Autodesk Inventor part; units mm, degrees
ref_plane "YZ Plane" through (0, 0, 0) normal (1, 0, 0) x (0, 1, 0)
ref_plane "XZ Plane" through (0, 0, 0) normal (0, 1, 0) x (-1, 0, 0)
ref_plane "XY Plane" through (0, 0, 0) normal (0, 0, 1) x (1, 0, 0)
sketch "Sketch1" plane through (0, 0, 0) normal (1, 0, 0) x (0, 1, 0)
  line L0 (95.25, 812.8) -> (44.45, 812.8) construction
  line L1 (44.45, 812.8) -> (44.45, 0) construction
  line L2 (44.45, 0) -> (95.25, 0) construction
  line L3 (95.25, 0) -> (95.25, 812.8) construction
  line L4 (95.25, 0) -> (44.45, 0) construction
  line L5 (44.45, 25.4) -> (95.25, 25.4) construction
  circle A0 centre (190.5, 0) radius 50.8 construction
  circle A1 centre (95.25, 279.4) radius 25.4 construction
  circle A2 centre (274.9493, 279.9916) radius 9.525 construction
  circle A3 centre (274.9493, 279.9916) radius 25.4 construction
  circle A4 centre (274.9493, 279.9916) radius 31.75 construction
  circle A5 centre (609.6, 438.15) radius 50.8 construction
  circle A6 centre (274.9493, 279.9916) radius 30.48 construction
  circle A7 centre (587.8333, 365.125) radius 25.4 construction
  circle A8 centre (587.8333, 511.175) radius 25.4 construction
  line L6 (587.8333, 485.775) -> (587.8333, 390.525) construction
  circle A9 centre (490.3356, 512.7625) radius 14.351
  circle A10 centre (392.825, 512.7625) radius 14.351
  circle A11 centre (490.3356, 363.5375) radius 14.351
  line L7 (587.8333, 511.175) -> (490.3356, 512.7625) construction
  line L8 (587.8333, 365.125) -> (490.3356, 363.5375) construction
  circle A12 centre (490.3356, 512.7625) radius 25.4 construction
  circle A13 centre (490.3356, 363.5375) radius 25.4 construction
  line L9 (490.3356, 487.3625) -> (490.3356, 388.9375) construction
  circle A14 centre (392.825, 512.7625) radius 25.4 construction
  circle A15 centre (392.825, 363.5375) radius 25.4 construction
  circle A16 centre (392.825, 363.5375) radius 14.351
  line L10 (490.3356, 512.7625) -> (392.825, 512.7625) construction
  line L11 (490.3356, 363.5375) -> (392.825, 363.5375) construction
  line L12 (392.825, 487.3625) -> (392.825, 388.9375) construction
  circle A17 centre (295.3189, 511.8309) radius 25.4 construction
  circle A18 centre (295.3189, 362.6059) radius 25.4 construction
  circle A19 centre (203.1597, 479.9719) radius 25.4 construction
  circle A20 centre (295.3189, 511.8309) radius 14.351
  circle A21 centre (295.3189, 362.6059) radius 14.351
  circle A22 centre (203.1597, 479.9719) radius 14.351
  line L13 (392.825, 512.7625) -> (295.3189, 511.8309) construction
  line L14 (392.825, 363.5375) -> (295.3189, 362.6059) construction
  line L15 (295.3189, 486.4309) -> (295.3189, 388.0059) construction
  line L16 (295.3189, 511.8309) -> (203.1597, 479.9719) construction
  circle A23 centre (123.1487, 424.2353) radius 25.4 construction
  circle A24 centre (123.1487, 424.2353) radius 14.351
  line L17 (203.1597, 479.9719) -> (123.1487, 424.2353) construction
  circle A25 centre (95.25, 279.4) radius 14.351
  line L18 (609.6, 355.6) -> (44.45, 355.6) construction
  line L19 (44.45, 355.6) -> (44.45, 330.2) construction
  line L20 (44.45, 330.2) -> (609.6, 330.2) construction
  line L21 (609.6, 330.2) -> (609.6, 355.6) construction
  line L22 (95.25, 241.3) -> (44.45, 241.3) construction
  line L23 (44.45, 241.3) -> (44.45, 215.9) construction
  line L24 (44.45, 215.9) -> (95.25, 215.9) construction
  line L25 (95.25, 215.9) -> (95.25, 241.3) construction
  circle A26 centre (244.475, 279.4) radius 25.4 construction
  circle A27 centre (244.475, 279.4) radius 14.351
  line L26 (218.8463, 459.9947) -> (279.6322, 382.5831) construction
  circle A28 centre (274.9493, 279.9916) radius 8.89 construction
  circle A29 centre (288.401, 252.6405) radius 21.59 construction
  circle A30 centre (244.475, 279.4) radius 21.59 construction
  circle A31 centre (288.401, 252.6405) radius 14.351
  circle A32 centre (587.8333, 511.175) radius 14.351
  circle A33 centre (587.8333, 365.125) radius 14.351
  line L27 (95.25, 647.7) -> (609.6, 647.7) construction
  line L28 (609.6, 647.7) -> (609.6, 622.3) construction
  line L29 (609.6, 622.3) -> (95.25, 622.3) construction
  line L30 (95.25, 622.3) -> (95.25, 647.7) construction
  circle A34 centre (600.5333, 552.45) radius 3.2639
  circle A35 centre (600.5333, 552.45) radius 6.35 construction
  circle A36 centre (600.5333, 336.55) radius 3.2639
  circle A37 centre (600.5333, 336.55) radius 6.35 construction
  circle A38 centre (114.3, 552.45) radius 3.2639
  circle A39 centre (114.3, 552.45) radius 6.35 construction
  line L31 (595.3031, 535.4518) -> (598.6659, 546.3808) construction
  circle A40 centre (63.5, 264.8503) radius 3.2639
  circle A41 centre (63.5, 264.8503) radius 6.35 construction
  line L32 (337.9424, 330.2) -> (600.5333, 330.2)
  circle A42 centre (288.401, 252.6405) radius 24.13 construction
  circle A43 centre (244.475, 279.4) radius 24.13 construction
  line L33 (72.1591, 268.8184) -> (69.2727, 267.4957) construction
  line L34 (609.6, 342.9) -> (44.45, 342.9) construction
  line L35 (265.0822, 266.8462) -> (267.7937, 265.1944) construction
  circle A44 centre (318.8924, 273.2978) radius 3.2639
  circle A45 centre (253.4257, 241.1003) radius 3.2639
  line L36 (95.25, 558.8) -> (44.45, 558.8) construction
  line L37 (44.45, 558.8) -> (44.45, 533.4) construction
  line L38 (44.45, 533.4) -> (95.25, 533.4) construction
  line L39 (95.25, 533.4) -> (95.25, 558.8) construction
  line L40 (114.3, 558.8) -> (600.5333, 558.8)
  line L41 (108.0468, 553.5545) -> (57.2468, 265.9549)
  line L42 (285.1949, 228.7245) -> (62.6563, 258.5566)
  circle A46 centre (318.8924, 273.2978) radius 6.35 construction
  circle A47 centre (253.4257, 241.1003) radius 6.35 construction
  arc A48 (114.3, 558.8) -> (108.0468, 553.5545) centre (114.3, 552.45) ccw
  arc A49 (57.2468, 265.9549) -> (62.6563, 258.5566) centre (63.5, 264.8503) ccw
  line L43 (312.6148, 274.2541) -> (306.3372, 275.2103) construction
  line L44 (313.6352, 269.7362) -> (308.3781, 266.1746) construction
  line L45 (259.4559, 243.09) -> (265.4861, 245.0797) construction
  line L46 (256.5005, 246.6562) -> (259.5753, 252.2121) construction
  line L47 (325.2424, 317.5) -> (325.2424, 273.2978)
  arc A50 (337.9424, 330.2) -> (325.2424, 317.5) centre (337.9424, 317.5) ccw
  line L48 (324.5494, 270.4133) -> (309.8976, 241.6792)
  arc A51 (324.5494, 270.4133) -> (325.2424, 273.2978) centre (318.8924, 273.2978) ccw
  arc A52 (285.1949, 228.7245) -> (309.8976, 241.6792) centre (288.401, 252.6405) ccw
  circle A53 centre (431.8, 342.9) radius 3.2639
  circle A54 centre (457.2, 342.9) radius 3.2639
  circle A55 centre (520.7, 342.9) radius 3.2639
  circle A56 centre (546.1, 342.9) radius 3.2639
  line L49 (606.8833, 552.45) -> (606.8833, 336.55)
  arc A57 (606.8833, 552.45) -> (600.5333, 558.8) centre (600.5333, 552.45) ccw
  arc A58 (600.5333, 330.2) -> (606.8833, 336.55) centre (600.5333, 336.55) ccw
  circle A59 centre (184.15, 304.8) radius 3.2639
  circle A60 centre (158.75, 304.8) radius 3.2639
  circle A61 centre (133.35, 304.8) radius 3.2639
  circle A62 centre (133.35, 279.4) radius 3.2639
  circle A63 centre (158.75, 279.4) radius 3.2639
  circle A64 centre (184.15, 279.4) radius 3.2639
  circle A65 centre (289.5545, 295.8051) radius 21.59 construction
  line L50 (313.8542, 277.163) -> (306.6842, 282.6636) construction
  circle A66 centre (289.5545, 295.8051) radius 14.351
  circle A67 centre (267.3295, 321.0778) radius 3.2639
  circle A68 centre (267.3295, 321.0778) radius 6.35 construction
  circle A69 centre (289.5545, 295.8051) radius 24.13 construction
  line L51 (271.5229, 316.3094) -> (273.6196, 313.9252) construction
  circle A70 centre (502.1083, 584.2) radius 3.2639
  circle A71 centre (349.7083, 584.2) radius 3.2639
  circle A72 centre (197.3083, 584.2) radius 3.2639
  circle A73 centre (502.1083, 584.2) radius 12.7 construction
  circle A74 centre (197.3083, 584.2) radius 12.7 construction
  line L52 (509.8384, 594.2765) -> (556.0833, 558.8)
  line L53 (502.1083, 596.9) -> (197.3083, 596.9)
  line L54 (191.9353, 595.7074) -> (111.6135, 558.2037)
  arc A75 (509.8384, 594.2765) -> (502.1083, 596.9) centre (502.1083, 584.2) ccw
  arc A76 (197.3083, 596.9) -> (191.9353, 595.7074) centre (197.3083, 584.2) ccw
  point P0 (0, 0)
  point P1 (241.139, 234.6303)
  point P2 (100.4185, 253.4945)
  dimension "d9" = 50.8
  dimension "d38" = 50.8
  dimension "d53" = 50.8
  dimension "d178" = 43.18
  dimension "d183" = 2.54
  dimension "d1" = 812.8
  dimension "d2" = 44.45
  dimension "d4" = 25.4
  dimension "d5" = 101.6
  dimension "d6" = 95.25
  dimension "d8" = 50.8
  dimension "d14" = 50.8
  dimension "d15" = 63.5
  dimension "d21" = 19.05
  dimension "d29" = 438.15
  dimension "d30" = 514.35
  dimension "d36" = 60.96
  dimension "d39" = 50.8
  dimension "d41" = 95.25
  dimension "d45" = 28.702
  dimension "d47" = 97.5106
  dimension "d48" = 98.425
  dimension "d56" = 25.4
  dimension "d73" = 50.8
  dimension "d74" = 25.4
  dimension "d75" = 215.9
  dimension "d78" = 279.4
  dimension "d80" = 149.225
  dimension "d81" = 97.5106
  dimension "d82" = 147.4978
  dimension "d83" = 17.78
  dimension "d85" = 43.18
  dimension "d92" = 330.2
  dimension "d100" = 514.35
  dimension "d107" = 25.4
  dimension "d108" = 514.35
  dimension "d109" = 266.7
  dimension "d115" = 6.5278
  dimension "d116" = 12.7
  dimension "d122" = 2.54
  dimension "d123" = 2.54
  dimension "d128" = 3.175
  dimension "d134" = 3.175
  dimension "d135" = 194.9958
  dimension "d136" = 6.5278
  dimension "d137" = 25.4
  dimension "d138" = 533.4
  dimension "d139" = 19.05
  dimension "d140" = 19.05
  dimension "d141" = 12.7
  dimension "d142" = 6.35
  dimension "d143" = 12.7
  dimension "d144" = 43.18
  dimension "d149" = 25.4
  dimension "d151" = 6.5278
  dimension "d157" = 25.4
  dimension "d158" = 63.5
  dimension "d159" = 12.7
  dimension "d161" = 11.4347
  dimension "d163" = 44.45
  dimension "d164" = 38.1
  dimension "d166" = 336.55
  dimension "d167" = 25.4
  dimension "d168" = 6.5278
  dimension "d169" = 25.4
  dimension "d170" = 25.4
  dimension "d173" = 25.4
  dimension "d174" = 38.1
  dimension "d175" = 25.4
extrude "Extrusion2" add sketch "Sketch1" along normal blind 6.35
properties part number "INDX_011_SecondPlate" material "Polycarbonate, Clear"
The model under review builds one solid part; all positions refer to its coordinate system, in mm. Round coordinates to 2 decimals unless told otherwise and drop trailing zeros. Write each loop counter-clockwise with the first axis right and the second up, starting at its lowest first coordinate (ties: lowest second). Pieces come first, ordered by that corner, then holes. Notation, with made-up numbers: M 49,8 L 56,8 A13 ccw 56,15 Z; hole C -4.5,74 d3. An arc over 180 degrees is marked long. Use a Markdown table: item, result. Add a question column.
Q1. We need section A-A, the plane y = 485.5. State the section outline as (x, z) points, plus the area to 3 significant figures.
Q2. The part is to be moulded in two halves that separate along Z. For faces 1 (the face through (6.35, 328, 415)), 2 (the face through (3.131, 175.483, 243.432)), 3 (the face through (3.13, 302.81, 301.3)), 4 (the face through (3.1, 152.3, 577.2)), say which applies: pulls with the +Z half, pulls with the -Z half, needs draft (parallel to the pull), parting line crosses it, or undercut.
Q3. To check wall thickness, follow line 1 (Y direction, x = 5.5, z = 278.5); line 2 (Y direction, x = 4, z = 304.8); line 3 (Z direction, x = 2, y = 405). State the ranges of each line that lie inside material, in increasing order.
Q4. We need section D-D, the plane y = 413.5. State the section outline as (x, z) points.
Q5. Insertion check: pin 1 (5 mm diameter, centred on y = 502.11, z = 584.2, fed in from +X); pin 2 (8 mm diameter, centred on y = 234, z = 471, fed in from -X). Each pin has a flat end and moves straight along its axis. Give the tip position at first contact, or say it passes through.
Q6. We need section B-B, the plane y = 95.25. State the section outline as (x, z) points, plus the area to 3 significant figures.
Q7. We need section C-C, the plane x = 3.75. Count the separate pieces of the cut face and the enclosed holes in it, plus the area to 3 significant figures.
Findings below:
| question | item | result |
|---|---|---|
| 1 | outline | M 0,330.2 L 6.35,330.2 L 6.35,350.03 L 0,350.03 Z; M 0,377.05 L 6.35,377.05 L 6.35,499.25 L 0,499.25 Z; M 0,526.27 L 6.35,526.27 L 6.35,596.9 L 0,596.9 Z |
| 1 | area | 1,350 mm² |
| 2 | face 1 | needs draft |
| 2 | face 2 | pulls with the -Z half |
| 2 | face 3 | undercut |
| 2 | face 4 | pulls with the +Z half |
| 3 | line 1 | y = 59.46 to 80.93, 109.57 to 130.21, 136.49 to 155.61, 161.89 to 181.01, 187.29 to 230.15, 258.8 to 325.24 |
| 3 | line 2 | y = 64.11 to 130.09, 136.61 to 155.49, 162.01 to 180.89, 187.41 to 278.37, 300.74 to 325.24 |
| 3 | line 3 | z = 330.2 to 355.94, 371.13 to 505.17, 520.36 to 596.9 |
| 4 | outline | M 0,330.2 L 6.35,330.2 L 6.35,596.9 L 0,596.9 Z |
| 5 | pin 1 | passes through |
| 5 | pin 2 | stops at x = 0 |
| 6 | outline | M 0,254.19 L 6.35,254.19 L 6.35,265.05 L 0,265.05 Z; M 0,293.75 L 6.35,293.75 L 6.35,481.11 L 0,481.11 Z |
| 6 | area | 1,260 mm² |
| 7 | separate pieces | 1 |
| 7 | enclosed holes | 34 |
| 7 | area | 146,000 mm² |
